from build123d import *

# Parameters (mm, degrees)
EXTRUDE1_DEPTH                              = 80
CBORE_FOR_M5_HEX_HEAD_CAP_SCREW1_AT_2_COUNT = 2
CBORE_FOR_M5_HEX_HEAD_CAP_SCREW1_AT_2_PITCH = 25
CBORE_FOR_M5_HEX_HEAD_CAP_SCREW1_AT_3_COUNT = 2
CBORE_FOR_M5_HEX_HEAD_CAP_SCREW1_AT_3_PITCH = 50


with BuildPart() as part:
    # Sketch1 → Extrude1 (new body)
    with BuildSketch(Plane.XY):
        Polygon((-13, 0), (-4, 0), (-4, -2.5), (-7.5, -2.5), (-7.5, -4.5), (-5.5, -6.5), (5.5, -6.5), (7.5, -4.5), (7.5, -2.5), (4, -2.5), (4, 0), (13, 0), (13, 5), (-13, 5), align=None)
    extrude(amount=EXTRUDE1_DEPTH)

    # Sketch3 → CBORE for M5 Hex Head Cap Screw1 (revolve, cut)
    with BuildSketch(Plane(origin=(0, 5, 65), x_dir=(0, 0, 1), z_dir=(1, 0, 0))):
        Polygon((0, 0), (0, 11.5), (1.4, 11.5), (2.1, 11.5), (2.1, 10), (1.4, 10), (1.4, 1.5), (2.1, 1.5), (2.1, 0), align=None)
    cbore_for_m5_hex_head_cap_screw1 = revolve(axis=Axis((0, 11.35, 65), (0, -1, 0)), mode=Mode.SUBTRACT)

    # CBORE for M5 Hex Head Cap Screw1 at 2: CBORE for M5 Hex Head Cap Screw1 ×2
    with Locations(*[(0, 0, -i * CBORE_FOR_M5_HEX_HEAD_CAP_SCREW1_AT_2_PITCH) for i in range(1, CBORE_FOR_M5_HEX_HEAD_CAP_SCREW1_AT_2_COUNT)]):
        add(cbore_for_m5_hex_head_cap_screw1, mode=Mode.SUBTRACT)

    # CBORE for M5 Hex Head Cap Screw1 at 3: CBORE for M5 Hex Head Cap Screw1 ×2
    with Locations(*[(0, 0, -i * CBORE_FOR_M5_HEX_HEAD_CAP_SCREW1_AT_3_PITCH) for i in range(1, CBORE_FOR_M5_HEX_HEAD_CAP_SCREW1_AT_3_COUNT)]):
        add(cbore_for_m5_hex_head_cap_screw1, mode=Mode.SUBTRACT)


solid = part.part
Design review of the part built by this model. Coordinates are the model's own, in mm. A direction names the side the tool comes from. Round coordinates to 2 decimals unless told otherwise and drop trailing zeros. Order: outer loops, then holes, each group sorted by start corner. A loop starts at its lowest first (then second) coordinate and runs counter-clockwise, first axis right, second up. Notation, with made-up numbers: M -24,61 L 5,61 A20 ccw 5,66 Z; hole C -22,57.5 d8. An arc over 180 degrees is marked long. Answer as CSV lines item,"result". Start each with the question number.
1) Tool access review of faces 1 (the face through (-9, 0, 39)), 2 (the face through (-0.631, -5.74, 17.003)), 3 (the face through (4, -1, 39)): name each direction out of +Z, -Z, +X, -X, +Y, -Y from which nothing blocks a thin tool from reaching the whole face with its end or side.
2) Add section C-C (x = 0). Give the number of separate pieces and of enclosed holes in the cut face, then the cut area to 3 significant figures.
3) Add section D-D (z = 74). Give the boundary of the cut face in (x, y), then the cut area to 3 significant figures.
4) For pin 1 Ø2 at (x, z) = (-0.5, 15) entering from +Y; pin 2 Ø4.5 at (x, z) = (0, 14) entering from -Y; pin 3 Ø1.3 at (x, z) = (0.5, 64) entering from -Y; pin 4 Ø0.8 at (y, z) = (-1.5, 27.5) entering from +X, all flat-tipped, find the tip position at first contact; note any pin that passes through.
5) Add section B-B (y = -1.5). Give the boundary of the cut face in (x, z).
6) The part is to be moulded in two halves that separate along Y. For faces 4 (the face through (6, -6, 39)), 5 (the face through (3, 5, 39)), 6 (the face through (-4, -1, 39)), 7 (the face through (0.54, -0.69, 41.29)), say which applies: +Y half, -Y half, draft (parallel to the pull), parting line (faces both ways), or undercut.
7) Wall thickness on line 1 along Z through (x, y) = (0, 4.55); line 2 along Z through (x, y) = (0, 1.75); line 3 along X through (y, z) = (4.05, 15): over which ranges is each line inside the solid? List them lowest first. Write a range as [from, to].
8) Add section A-A (z = 40). Give the boundary of the cut face in (x, y), then the cut area to 3 significant figures.
Resolved:
1,face 1,"+Z, -Z, -X"
1,face 2,"-Y"
1,face 3,"+Z, -Z, +X"
2,separate pieces,"4"
2,enclosed holes,"0"
2,area,"811 mm^2"
3,outline,"M -13,0 L -4,0 L -4,-2.5 L -7.5,-2.5 L -7.5,-4.5 L -5.5,-6.5 L 5.5,-6.5 L 7.5,-4.5 L 7.5,-2.5 L 4,-2.5 L 4,0 L 13,0 L 13,5 L -13,5 Z"
3,area,"206 mm^2"
4,pin 1,"y = 3.5"
4,pin 2,"y = -6.5"
4,pin 3,"y = -5"
4,pin 4,"x = 4"
5,outline,"M -4,0 L 4,0 L 4,80 L -4,80 Z; hole C 0,15 d2.8; hole C 0,40 d2.8; hole C 0,65 d2.8"
6,face 4,"-Y half"
6,face 5,"+Y half"
6,face 6,"undercut"
6,face 7,"draft"
7,line 1,"[0, 12.9], [17.1, 37.9], [42.1, 62.9], [67.1, 80]"
7,line 2,"[0, 13.6], [16.4, 38.6], [41.4, 63.6], [66.4, 80]"
7,line 3,"[-13, -2.1], [2.1, 13]"
8,outline,"M -13,0 L -4,0 L -4,-2.5 L -7.5,-2.5 L -7.5,-4.5 L -5.5,-6.5 L -2.1,-6.5 L -2.1,-5 L -1.4,-5 L -1.4,3.5 L -2.1,3.5 L -2.1,5 L -13,5 Z; M 1.4,-5 L 2.1,-5 L 2.1,-6.5 L 5.5,-6.5 L 7.5,-4.5 L 7.5,-2.5 L 4,-2.5 L 4,0 L 13,0 L 13,5 L 2.1,5 L 2.1,3.5 L 1.4,3.5 Z"
8,area,"170 mm^2"
